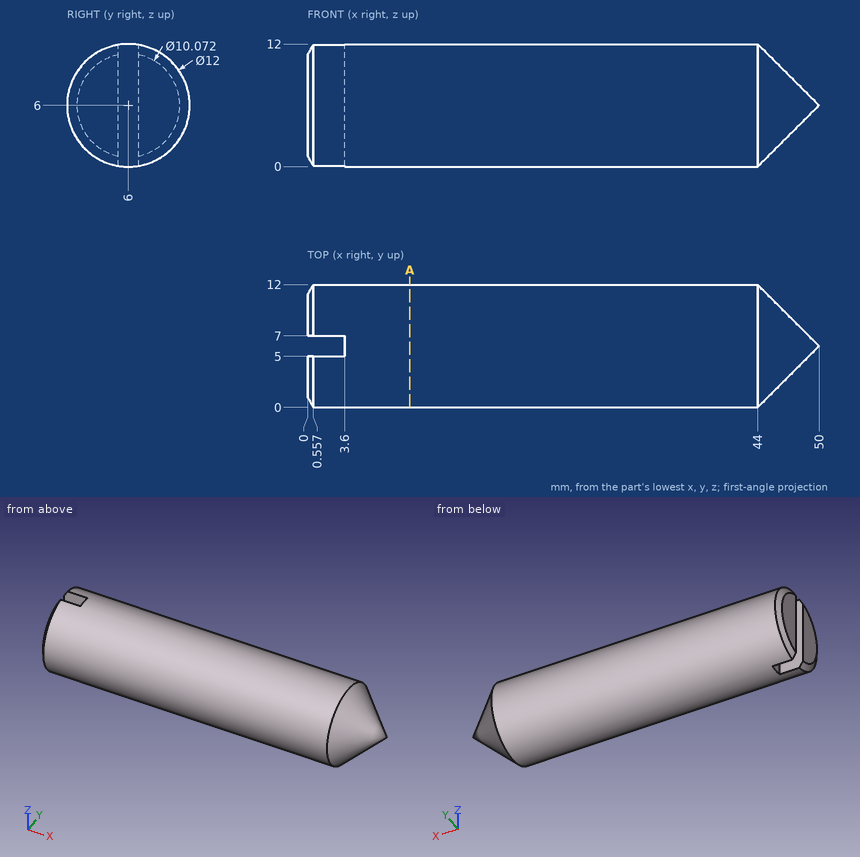
Here's the drawing with two shaded views (mm, measured from the low corner). I have some questions. Round coordinates to 2 decimals unless told otherwise and drop trailing zeros. Order: outer loops, then holes, each group sorted by start corner. A loop starts at its lowest first (then second) coordinate and runs counter-clockwise, first axis right, second up. Notation, with made-up numbers: (88.25, 79) -> (108.25, 79) arc R33 ccw to (108.25, 107) -> close; hole circle Ø3 at (9.5, -34). An arc over 180 degrees is marked (long way). Return JSON: item names as keys, results as strings.
Q1. If we section it at A-A on x = 10: List the corners of the cut face in (y, z) for me, plus the area to 3 significant figures.
Filled sheet:
{"outline": "circle Ø12 at (6, 6)", "area": "113 mm^2"}
Q2. I need wall thicknesses on line 1 along Z through (x, y) = (22, 7) (1 decimal); line 2 along Y through (x, z) = (21, 9.25) (1 decimal); line 3 along Y through (x, z) = (39, 4.5). Which ranges of each line are inside material? Lowest first, please. Write a range as from..to.
Filled sheet:
{"line 1": "z = 0.1..11.9", "line 2": "y = 1..11", "line 3": "y = 0.19..11.81"}
Q3. For pin 1 Ø0.6 at (y, z) = (6, 6) entering from -X; pin 2 Ø1.1 at (x, z) = (2.5, 4.5) entering from +Y, each with a flat end and sliding along its axis, tell me the tip position at first contact or that it passes through.
Filled sheet:
{"pin 1": "stops at x = 3.6", "pin 2": "stops at y = 11.92"}
